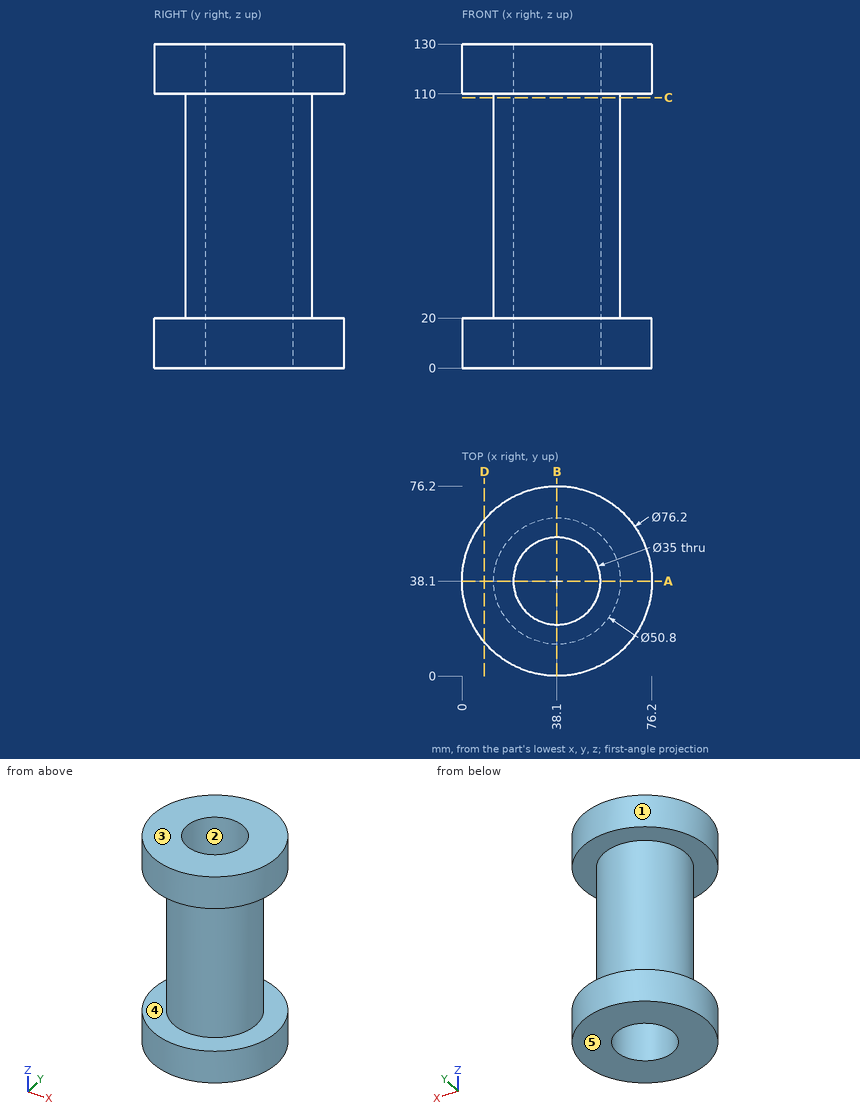
Part print with two shaded views. Sizes in mm from the minimum x, y, z corner. A direction names the side the tool comes from. Coordinates: 2 decimals unless noted, no trailing zeros. Write each loop counter-clockwise with the first axis right and the second up, starting at its lowest first coordinate (ties: lowest second). Pieces come first, ordered by that corner, then holes. Notation, with made-up numbers: (19.25, 85.5) - (26.25, 85.5) arc R19 ccw to (26.25, 113.5) - close; hole circle Ø6 at (34.25, 66). An arc over 180 degrees is marked (long way). Put each result on its own line as item: value.
1. Probe line 1 along Y through (x, z) = (38.1, 72.5); line 2 along Z through (x, y) = (20, 5.5). List the from-to ranges inside material, lowest first. Write a range as [from, to].
Final values:
line 1: y = [12.7, 20.6], [55.6, 63.5]
line 2: z = [0, 20], [110, 130]
2. 3-axis set-ups, long thin cutter, end or side, ignore diameter. For the marked faces 4 and 5: which of +Z, -Z, +X, -X, +Y, -Y reach the whole face in a straight line?
Final values:
face 4: none
face 5: -Z, +X, -X, +Y, -Y
3. Band-saw the part on A-A (y = 38.1). Write the cut outline in (x, z), then the cut area to 3 significant figures.
Final values:
outline: (0, 0) - (20.6, 0) - (20.6, 130) - (0, 130) - (0, 110) - (12.7, 110) - (12.7, 20) - (0, 20) - close; (55.6, 0) - (76.2, 0) - (76.2, 20) - (63.5, 20) - (63.5, 110) - (76.2, 110) - (76.2, 130) - (55.6, 130) - close
area: 3,070 mm²
4. Band-saw the part on D-D (x = 9). Write the cut outline in (y, z).
Final values:
outline: (13.51, 0) - (62.69, 0) - (62.69, 20) - (13.51, 20) - close; (13.51, 110) - (62.69, 110) - (62.69, 130) - (13.51, 130) - close
5. Band-saw the part on C-C (z = 108.5). Write the cut outline in (x, y), then the cut area to 3 significant figures.
Final values:
outline: circle Ø50.8 at (38.1, 38.1); hole circle Ø35 at (38.1, 38.1)
area: 1,060 mm²
6. Flat gauge pins, fed straight in: pin 1 Ø4 at (y, z) = (62.5, 42.5) entering from -X (3 decimals); pin 2 Ø1.5 at (y, z) = (64.5, 116.5) entering from +X; pin 3 Ø10 at (y, z) = (58, 82.5) entering from -X; pin 4 Ø10 at (x, y) = (21, 32) entering from -Z. Where does each tip first touch, or does it go through?
Final values:
pin 1: stops at x = 26.125
pin 2: stops at x = 66.27
pin 3: stops at x = 17.53
pin 4: stops at z = 0
7. Two-plate mould, pull along Y, no slides. Class the marked faces 1, 2 and 3: +Y half, -Y half, draft (parallel to the pull), parting line (faces both ways), or undercut.
Final values:
face 1: parting line
face 2: undercut
face 3: draft
